CAD build for the part. Positions are in the model's coordinates, mm. A direction names the side the tool comes from. Coordinates: 2 decimals unless noted, no trailing zeros. Order: outer loops, then holes, each group sorted by start corner. A loop starts at its lowest first (then second) coordinate and runs counter-clockwise, first axis right, second up.
from build123d import *

# Parameters (mm, degrees)
F_1_4_20_TAPPED_HOLE1_D = 5.1054


with BuildPart() as part:
    # Sketch1 → Revolve1 (revolve)
    with BuildSketch(Plane.XY):
        Polygon((0, 0), (0, 6.35), (4.7625, 6.35), (4.7625, 12.7), (14.2875, 12.7), (14.2875, 6.35), (19.05, 6.35), (19.05, 0), align=None)
    revolve(axis=Axis((19.05, 0, 0), (-1, 0, 0)))

    # 1/4-20 Tapped Hole1 (through all)
    with Locations(Plane(origin=(19.05, 0, 0), x_dir=(0, 0, -1), z_dir=(1, 0, 0))):
        with Locations((0, 0)):
            Hole(F_1_4_20_TAPPED_HOLE1_D / 2)


solid = part.part
1) Drill centre lines: probe 1 along Y at (x, z) = (6, 0); probe 2 along X at (y, z) = (-3, 6); probe 3 along Y at (x, z) = (4.5, 0). Where is each one in solid material? Low to high.
2) Two-plate mould, pull along Y, no slides. Class faces 1 (the flat face through (0, -3, 0)), 2 (the cylindrical face through (2.41, -1.38, 6.2)), 3 (the cylindrical face through (9.392, 0.767, 2.435)): released by +Y, released by -Y, zero draft, split by the parting line, or undercut.
3) Slice it at C-C (x = 10). List the corners of the cut face in (y, z), plus the area to 3 significant figures.
4) Which spindle directions (+Z, -Z, +X, -X, +Y, -Y) get a long thin tool onto all of the face, cutting with end or side? Do faces 4 (the flat face through (4.762, -3, -6)), 5 (the cylindrical face through (9.59, -2.75, 12.4)), 6 (the cylindrical face through (16.7, -1.38, 6.2)). Say none if no direction does.
5) Slice it at A-A (y = 0). List the corners of the cut face in (x, z).
6) Pin check, flat tips, straight feed: P1, Ø6, axis at y = -6.5, z = 8, coming from the -X side; P2, Ø1, axis at x = 3, z = 5.5, coming from the +Y side; P3, Ø3, axis at x = 12, z = 9, coming from the +Y side. Stop position of each tip, or through.
7) Slice it at D-D (z = -5.75). List the corners of the cut face in (x, y).
Worked out:
1. probe 1: y = -12.7 to -2.55, 2.55 to 12.7
1. probe 2: x = 4.76 to 14.29
1. probe 3: y = -6.35 to -2.55, 2.55 to 6.35
2. face 1: zero draft
2. face 2: split by the parting line
2. face 3: undercut
3. outline: circle Ø25.4 at (0, 0); hole circle Ø5.11 at (0, 0)
3. area: 486 mm2
4. face 4: -X
4. face 5: +X, -X
4. face 6: +X
5. outline: (0, -6.35) - (4.76, -6.35) - (4.76, -12.7) - (14.29, -12.7) - (14.29, -6.35) - (19.05, -6.35) - (19.05, -2.55) - (0, -2.55) - close; (0, 2.55) - (19.05, 2.55) - (19.05, 6.35) - (14.29, 6.35) - (14.29, 12.7) - (4.76, 12.7) - (4.76, 6.35) - (0, 6.35) - close
6. P1: stops at x = 4.76
6. P2: stops at y = 3.91
6. P3: stops at y = 10.25
7. outline: (0, -2.69) - (4.76, -2.69) - (4.76, -11.32) - (14.29, -11.32) - (14.29, -2.69) - (19.05, -2.69) - (19.05, 2.69) - (14.29, 2.69) - (14.29, 11.32) - (4.76, 11.32) - (4.76, 2.69) - (0, 2.69) - close
